from build123d import *

# Parameters (mm, degrees)
CROQUIS1_W              = 27.8
CROQUIS1_H              = 16
SALIENTE_EXTRUIR1_DEPTH = 4.8
REDONDEO1_R             = 2
SALIENTE_EXTRUIR2_START = 2.075
CROQUIS2_R              = 0.75
SALIENTE_EXTRUIR2_DEPTH = 0.8
SALIENTE_EXTRUIR3_DEPTH = 3.2
CROQUIS4_R              = 0.75
SALIENTE_EXTRUIR4_DEPTH = 0.8
CROQUIS5_R              = 1.625
CORTAR_EXTRUIR1_DEPTH   = 28.66604417
CROQUIS6_W              = 4.2
CROQUIS6_H              = 2.8
SALIENTE_EXTRUIR5_DEPTH = 3
REDONDEO2_R             = 1.4


with BuildPart() as part:
    # Croquis1 → Saliente-Extruir1 (new, symmetric)
    with BuildSketch(Plane(origin=(0, 0, 0), x_dir=(0, 0, -1), z_dir=(1, 0, 0))):
        Rectangle(CROQUIS1_W, CROQUIS1_H)
    extrude(amount=SALIENTE_EXTRUIR1_DEPTH, both=True)

    # Redondeo1
    redondeo1_edges = [part.edges().sort_by_distance(p)[0] for p in [
        (0, -8, -13.9),
        (0, -8, 13.9),
        (0, 8, 13.9),
        (0, 8, -13.9),
    ]]
    fillet(redondeo1_edges, radius=REDONDEO1_R)

    # Croquis2 → Saliente-Extruir2 (add)
    with BuildSketch(Plane(origin=(0, 0, 0), x_dir=(1, 0, 0), z_dir=(0, 1, 0)).offset(SALIENTE_EXTRUIR2_START)):
        Polygon((3.2, 13.9), (-3.2, 13.9), (-3.2, 17.3), (-2.4, 17.3), (-2.4, 22.6), (-1.5, 23.5), (1.5, 23.5), (2.4, 22.6), (2.4, 17.3), (3.2, 17.3), align=None)
        with Locations(Location((0, 20.5, 0), (0, 0, 270))):
            Circle(CROQUIS2_R, mode=Mode.SUBTRACT)
    saliente_extruir2 = extrude(amount=SALIENTE_EXTRUIR2_DEPTH)

    # Simetría1: Saliente-Extruir2 across plane
    add(saliente_extruir2.mirror(Plane.ZX))

    # Croquis3 → Saliente-Extruir3 (add, symmetric)
    with BuildSketch(Plane(origin=(0, 0, 0), x_dir=(0, 0, -1), z_dir=(1, 0, 0))):
        with BuildLine():
            Line((1.4, 8), (2.005248739, 10.258819045))
            ThreePointArc((2.005248739, 10.258819045), (2.362413136, 10.79335334), (2.971174565, 11))
            Line((2.971174565, 11), (4.703847577, 11))
            Line((4.703847577, 11), (4.703847577, 10.2))
            Line((4.703847577, 10.2), (2.971174565, 10.2))
            ThreePointArc((2.971174565, 10.2), (2.849422279, 10.158670668), (2.7779894, 10.051763809))
            Line((2.7779894, 10.051763809), (2.228220944, 8))
            Line((2.228220944, 8), (1.4, 8))
        make_face()
    extrude(amount=SALIENTE_EXTRUIR3_DEPTH, both=True)

    # Croquis4 → Saliente-Extruir4 (add)
    with BuildSketch(Plane(origin=(0, 11, 0), x_dir=(1, 0, 0), z_dir=(0, 1, 0))):
        Polygon((-2.4, 4.703847577), (-2.4, 10.003847577), (-1.5, 10.903847577), (1.5, 10.903847577), (2.4, 10.003847577), (2.4, 4.703847577), align=None)
        with Locations(Location((0, 7.903847577, 0), (0, 0, 270))):
            Circle(CROQUIS4_R, mode=Mode.SUBTRACT)
    extrude(amount=-SALIENTE_EXTRUIR4_DEPTH)

    # Croquis5 → Cortar-Extruir1 (cut, through all)
    with BuildSketch(Plane(origin=(4.8, 0, 0), x_dir=(0, 0, -1), z_dir=(1, 0, 0))):
        with Locations((-11.075, 5.325)):
            Circle(CROQUIS5_R)
        with Locations((11.125, -5.225)):
            Circle(CROQUIS5_R)
    extrude(amount=-CORTAR_EXTRUIR1_DEPTH, mode=Mode.SUBTRACT)

    # Croquis6 → Saliente-Extruir5 (add)
    with BuildSketch(Plane.XZ.offset(8)):
        with Locations((0, 9.5)):
            Rectangle(CROQUIS6_W, CROQUIS6_H)
    extrude(amount=SALIENTE_EXTRUIR5_DEPTH)

    # Redondeo2
    redondeo2_edges = [part.edges().sort_by_distance(p)[0] for p in [
        (0, -11, 8.1),
        (0, -11, 10.9),
    ]]
    fillet(redondeo2_edges, radius=REDONDEO2_R - 0.0001)  # a hair under: the kernel refuses the full size


solid = part.part
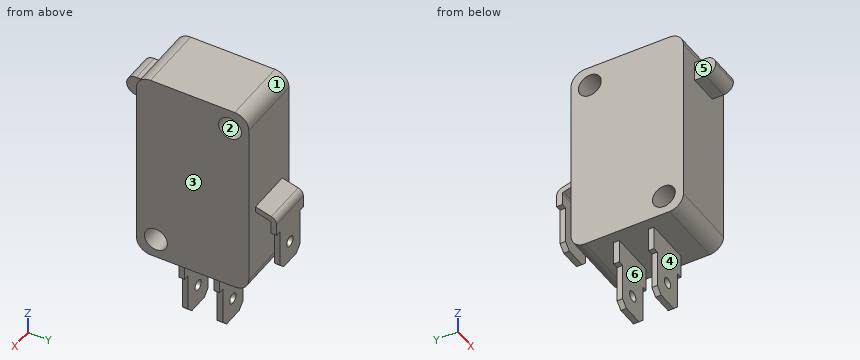
The model under review builds one solid part; all positions refer to its coordinate system, in mm. Face numbers are marked on the shaded views. A direction names the side the tool comes from. Give positions to 0.01 mm unless a question says otherwise; leave off trailing zeros. Write each loop counter-clockwise with the first axis right and the second up, starting at its lowest first coordinate (ties: lowest second). Pieces come first, ordered by that corner, then holes. Notation, with made-up numbers: M 42.5,78.25 L 92.5,78.25 A22 ccw 92.5,109.25 Z; hole C -4,69 d3. An arc over 180 degrees is marked long. One line per question, with ' | ' between items. Start each with the question number.
Item 1: We need section D-D on x = 0. Give the number of separate pieces and of enclosed holes in the cut face, plus the area to 3 significant figures.
Item 2: We need section B-B on z = -20.5. Write out the cut boundary in (x, y) (3 decimals).
Item 3: Draft analysis for pull direction Z (two halves, no side actions). For the marked faces 1, 2 and 3, state which applies: released by +Z, released by -Z, zero draft, split by the parting line, or undercut.
Item 4: For pin 1 (0.6 mm diameter, centred on x = 3, y = 2.5, fed in from -Z); pin 2 (0.6 mm diameter, centred on y = 2.5, z = -16, fed in from -X); pin 3 (3 mm diameter, centred on y = 2.5, z = -14, fed in from -X); pin 4 (1.3 mm diameter, centred on x = 1, y = -9, fed in from -Z), all flat-tipped, find the tip position at first contact; note any pin that passes through.
Item 5: For the marked faces 4, 5 and 6, list the 3-axis set-ups (+Z, -Z, +X, -X, +Y, -Y) from which the entire face can be reached by the end or side of a thin tool; tool diameter is ignored.
Item 6: We need section C-C on y = 1.5. Write out the cut boundary in (x, z).
Item 7: We need section A-A on z = -4. Write out the cut boundary in (x, y), plus the area to 3 significant figures.
Item 8: Wall thickness on line 1 (X direction, y = 2.4, z = -20.5); line 2 (Y direction, x = 2.5, z = -15) (3 decimals); line 3 (Y direction, x = -1.5, z = -4): over which ranges is each line inside the solid? List them lowest first. Write a range as from..to.
Results found:
1) separate pieces: 4 | enclosed holes: 2 | area: 453 mm2
2) outline: M -2.4,-2.875 L -0.75,-2.875 L -0.75,-2.075 L -2.4,-2.075 Z; M -2.4,2.075 L -0.75,2.075 L -0.75,2.875 L -2.4,2.875 Z; M 0.75,-2.875 L 2.4,-2.875 L 2.4,-2.075 L 0.75,-2.075 Z; M 0.75,2.075 L 2.4,2.075 L 2.4,2.875 L 0.75,2.875 Z
3) face 1: released by +Z | face 2: undercut | face 3: zero draft
4) pin 1: stops at z = -17.3 | pin 2: stops at x = -3.2 | pin 3: stops at x = -4.8 | pin 4: stops at z = 8.1
5) face 4: -Z, +X, -X, -Y | face 5: +Z, -Z, -X, -Y | face 6: -Z, +X, -X
6) outline: M -4.8,-13.9 L 4.8,-13.9 L 4.8,13.9 L -4.8,13.9 Z
7) outline: M -4.8,-8 L 4.8,-8 L 4.8,8 L -4.8,8 Z; M -3.2,10.2 L 3.2,10.2 L 3.2,11 L -3.2,11 Z | area: 159 mm2
8) line 1: x = -2.4..-0.75, 0.75..2.4 | line 2: y = -2.875..-2.075, 2.075..2.875 | line 3: y = -8..8, 10.2..11
